Check sheet for the modelled part. Datum: model origin and axes. Units: mm. Face numbers are marked on the shaded views. A direction names the side the tool comes from. Give positions to 0.01 mm unless a question says otherwise; leave off trailing zeros. Loops run counter-clockwise (first coordinate to the right, second up) from the corner with the lowest first, then second, coordinate; pieces in that order, holes last.
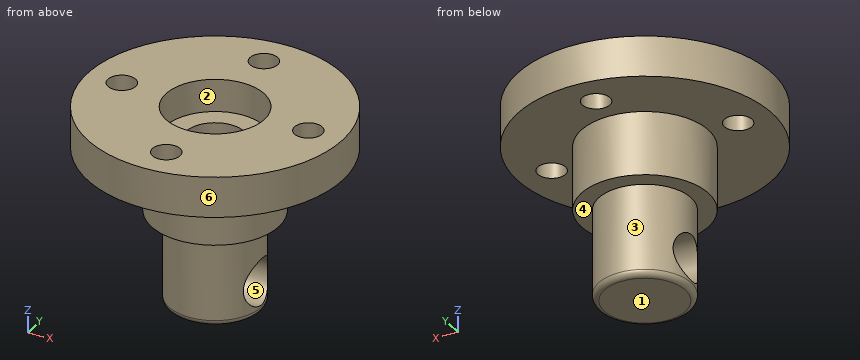
```python
from build123d import *

# Parameters (mm, degrees)
SKETCH_2_R               = 11
EXTRUDE_1_DEPTH          = 3.5
SKETCH_3_R               = 4.25
CUT_EXTRUDE_1_DEPTH      = 2.8
SKETCH_4_R               = 1.2
CUT_EXTRUDE_2_DEPTH      = 16.945218719
PATTERN_CIRCULAR_1_COUNT = 4
SKETCH_6_R               = 4
EXTRUDE_2_DEPTH          = 13.4
CUT_EXTRUDE1_DEPTH       = 21.531926359
CUT_EXTRUDE1_DEPTH_BACK  = 21.531926359
SKETCH1_R                = 2
SKETCH_15_R              = 5.5
EXTRUDE_3_DEPTH          = 5.5
FILLET_1_R               = 0.5
SKETCH_11_R              = 2.5
CUT_EXTRUDE_6_DEPTH      = 2.2


with BuildPart() as part:
    # 草图2 → 凸台-拉伸1 (new body)
    with BuildSketch(Plane.XY):
        Circle(SKETCH_2_R)
    extrude(amount=EXTRUDE_1_DEPTH)

    # 草图3 → 切除-拉伸1 (cut)
    with BuildSketch(Plane.XY.offset(3.5)):
        Circle(SKETCH_3_R)
    extrude(amount=-CUT_EXTRUDE_1_DEPTH, mode=Mode.SUBTRACT)

    # 草图4 → 切除-拉伸2 (cut, through all)
    with BuildSketch(Plane(origin=(0, 0, 0), x_dir=(-1, 0, 0), z_dir=(0, 0, -1))):
        with Locations((0, 8)):
            Circle(SKETCH_4_R)
    cut_extrude_2 = extrude(amount=-CUT_EXTRUDE_2_DEPTH, mode=Mode.SUBTRACT)

    # 阵列(圆周)1: 切除-拉伸2 ×4 about axis
    pattern_circular_1_axis = Axis((0, 0, 0), (0, 0, 1))
    for i in range(1, PATTERN_CIRCULAR_1_COUNT):
        add(cut_extrude_2.rotate(pattern_circular_1_axis, i * 360 / PATTERN_CIRCULAR_1_COUNT), mode=Mode.SUBTRACT)

    # 草图6 → 凸台-拉伸2 (add)
    with BuildSketch(Plane(origin=(0, 0, 0), x_dir=(-1, 0, 0), z_dir=(0, 0, -1))):
        with Locations(Location((0, 0, 0), (0, 0, 180))):
            Circle(SKETCH_6_R)
    extrude(amount=EXTRUDE_2_DEPTH)

    # Sketch1 → Cut-Extrude1 (cut, two sides: drawn at the far end of the back side and taken through both)
    with BuildSketch(Plane(origin=(0, 0, 0), x_dir=(0, 0, -1), z_dir=(1, 0, 0)).offset(-CUT_EXTRUDE1_DEPTH_BACK)):
        with Locations((10.7, 0)):
            Circle(SKETCH1_R)
    extrude(amount=CUT_EXTRUDE1_DEPTH + CUT_EXTRUDE1_DEPTH_BACK, mode=Mode.SUBTRACT)

    # 草图15 → 凸台-拉伸3 (add)
    with BuildSketch(Plane(origin=(0, 0, 0), x_dir=(-1, 0, 0), z_dir=(0, 0, -1))):
        with Locations(Location((0, 0, 0), (0, 0, 180))):
            Circle(SKETCH_15_R)
    extrude(amount=EXTRUDE_3_DEPTH)

    # 圆角1
    fillet_1_edges = [part.edges().sort_by_distance(p)[0] for p in [
        (-4, 0, -13.4),
    ]]
    fillet(fillet_1_edges, radius=FILLET_1_R)

    # 草图11 → 切除-拉伸6 (cut)
    with BuildSketch(Plane.XY.offset(0.7)):
        Circle(SKETCH_11_R)
    extrude(amount=-CUT_EXTRUDE_6_DEPTH, mode=Mode.SUBTRACT)


solid = part.part
```
(1) Gauge pin test, flat ends, axial feed: pin 1 Ø3 at (x, y) = (0, 8) entering from -Z; pin 2 Ø3 at (x, y) = (0, 0) entering from +Z; pin 3 Ø1.4 at (x, y) = (0, -8) entering from +Z; pin 4 Ø4 at (x, z) = (-2, -11) entering from -Y. Record the tip position at first contact, or that the pin passes through.
(2) Release check for a two-part mould opening along Y. For the marked faces 4, 5 and 6 record: pulls with the +Y half, pulls with the -Y half, needs draft (parallel to the pull), parting line crosses it, or undercut.
(3) Section check A-A on x = 0. Give the number of separate pieces and of enclosed holes in the cut face, plus the area to 3 significant figures.
(4) Access from +Z, -Z, +X, -X, +Y, -Y to the whole of each face (thin tool, end or side, straight path). Record for the marked faces 1, 2 and 3.
(5) Section check C-C on z = -1. Record the boundary of the cut face in (x, y), plus the area to 3 significant figures.
(6) Section check B-B on x = 8.5. Record the boundary of the cut face in (y, z).
(7) Section check D-D on y = -8. Record the boundary of the cut face in (x, z), plus the area to 3 significant figures.
(8) Material ranges on line 1 (Y direction, x = 0, z = 0.75); line 2 (Z direction, x = 7, y = 0.75); line 3 (Y direction, x = 2.25, z = -10.25), recorded low to high.
Computed values:
1. pin 1: stops at z = 0
1. pin 2: stops at z = -1.5
1. pin 3: passes through
1. pin 4: stops at y = -4
2. face 4: needs draft
2. face 5: undercut
2. face 6: parting line crosses it
3. separate pieces: 3
3. enclosed holes: 1
3. area: 136 mm2
4. face 1: -Z, +X, -X, +Y, -Y
4. face 2: +Z
4. face 3: -Z
5. outline: circle Ø11 at (0, 0); hole circle Ø5 at (0, 0)
5. area: 75.4 mm2
6. outline: (-6.98, 0) - (-1.09, 0) - (-1.09, 3.5) - (-6.98, 3.5) - close; (1.09, 0) - (6.98, 0) - (6.98, 3.5) - (1.09, 3.5) - close
7. outline: (-7.55, 0) - (-1.2, 0) - (-1.2, 3.5) - (-7.55, 3.5) - close; (1.2, 0) - (7.55, 0) - (7.55, 3.5) - (1.2, 3.5) - close
7. area: 44.4 mm2
8. line 1: y = -11 to -9.2, -6.8 to -4.25, 4.25 to 6.8, 9.2 to 11
8. line 2: z = 0 to 3.5
8. line 3: y = -3.31 to -1.95, 1.95 to 3.31
